```python
from build123d import *

# Parameters (mm, degrees)
F0_W          = 95.4247708432
F0_H          = 68.2654082775
F1_DEPTH      = 101.854
F3_DEPTH      = 90.424
F3_DEPTH_BACK = 11.43


with BuildPart() as f1:
    # F0 (on Front) → F1 (new body)
    with BuildSketch(Plane.XZ):
        with Locations((43.7975230161, -34.1327041388)):
            Rectangle(F0_W, F0_H)
    extrude(amount=F1_DEPTH)

    # F2 (on face) → F3 (join, two sides)
    with BuildSketch(Plane.XZ.offset(101.854)) as f3_sk:
        Polygon((-0.2897456373, 56.5875391827), (-6.536422763, 0), (91.5099084377, 0), align=None)
    extrude(amount=-F3_DEPTH)
    extrude(f3_sk.sketch, amount=F3_DEPTH_BACK)


solid = f1.part
```
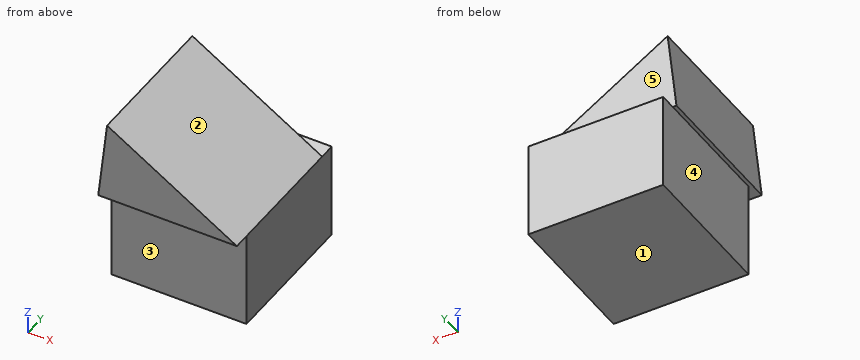
Could you check a few things on this model? Use its own coordinates, in mm. Face numbers are marked on the shaded views. A direction names the side the tool comes from. Coordinates: 2 decimals unless noted, no trailing zeros. Write each loop counter-clockwise with the first axis right and the second up, starting at its lowest first coordinate (ties: lowest second). Pieces come first, ordered by that corner, then holes. Notation, with made-up numbers: (35, 52.5) - (92, 52.5) arc R17 cw to (92, 72.5) - close; hole circle Ø3 at (-9, 34.25). An arc over 180 degrees is marked (long way). Use a Markdown table: item, result.
Q1. Which directions (+Z, -Z, +X, -X, +Y, -Y) give clear straight access to the entire face, cutting with the end or side of a thin tool? Please do the marked faces 1, 2, 3, 4 and 5.
Geometry check:
| item | result |
|---|---|
| face 1 | -Z, +X, -X, +Y, -Y |
| face 2 | +Z, +X, +Y, -Y |
| face 3 | -Z, +X, -X, -Y |
| face 4 | -Z, -X, +Y, -Y |
| face 5 | +Z, +X, -X, +Y |
Q2. I'm going to push flat-ended pins straight in: pin 1 Ø5 at (x, y) = (65.5, -65.5) entering from +Z; pin 2 Ø8 at (x, y) = (41, -15.5) entering from +Z; pin 3 Ø5 at (x, y) = (73, -83.5) entering from +Z. Where does each tip first touch, or does it pass through?
Geometry check:
| item | result |
|---|---|
| pin 1 | stops at z = 17.57 |
| pin 2 | stops at z = 33.6 |
| pin 3 | stops at z = 12.95 |
Q3. Please list where these lines run through material, in increasing order: L1, parallel to X at y = -49, z = -54.5; L2, parallel to Y at x = 37, z = -3; L3, parallel to Y at x = 10, z = 44.
Geometry check:
| item | result |
|---|---|
| L1 | x = -3.91 to 91.51 |
| L2 | y = -101.85 to 0 |
| L3 | y = -113.28 to -11.43 |
Q4. Imagine slicing it at C-C (y = -76.5). List the corners of the cut face in (x, z) for me, and give its area (3 significant figures).
Geometry check:
| item | result |
|---|---|
| outline | (-6.54, 0) - (-3.91, 0) - (-3.91, -68.27) - (91.51, -68.27) - (91.51, 0) - (-0.29, 56.59) - close |
| area | 9,290 mm2 |
Q5. Imagine slicing it at A-A (x = 18). List the corners of the cut face in (y, z) for me.
Geometry check:
| item | result |
|---|---|
| outline | (-113.28, 0) - (-101.85, 0) - (-101.85, -68.27) - (0, -68.27) - (0, 0) - (-11.43, 0) - (-11.43, 45.31) - (-113.28, 45.31) - close |
Q6. Imagine slicing it at B-B (z = -51). List the corners of the cut face in (x, y) for me.
Geometry check:
| item | result |
|---|---|
| outline | (-3.91, -101.85) - (91.51, -101.85) - (91.51, 0) - (-3.91, 0) - close |
Q7. Imagine slicing it at D-D (x = 66). List the corners of the cut face in (y, z) for me, and give its area (3 significant figures).
Geometry check:
| item | result |
|---|---|
| outline | (-113.28, 0) - (-101.85, 0) - (-101.85, -68.27) - (0, -68.27) - (0, 0) - (-11.43, 0) - (-11.43, 15.72) - (-113.28, 15.72) - close |
| area | 8,550 mm2 |
